Input: part model. Units: mm. Frame: model coordinates. Round coordinates to 2 decimals unless told otherwise and drop trailing zeros. Loops run counter-clockwise (first coordinate to the right, second up) from the corner with the lowest first, then second, coordinate; pieces in that order, holes last. Notation, with made-up numbers: M 58,-6 L 65,-6 A32 cw 65,27 Z; hole C 66,20 d7. An arc over 180 degrees is marked long. Use one line per item in the form item = value. Start each with the question number.
Q1. Mould query, pull axis X, two halves, no side actions, for faces 1 (the flat face through (61, 31, 27)), 2 (the cylindrical face through (66.96, 32.88, 31.93)), 3 (the flat face through (61, 31, 37)). Classes: pulls with the +X half, pulls with the -X half, needs draft (parallel to the pull), parting line crosses it, or undercut.
Q2. Ray query, line 1 along Z through (x, y) = (57.5, 33.25); line 2 along Y through (x, z) = (59.25, 34.25); line 3 along X through (y, z) = (30.25, 30). Return the intervals inside material, ascending.
Q3. Section query A-A, the plane y = 31. Output: boundary loops of the cut face in (x, z).
Q4. Section query B-B, the plane x = 61. Output: boundary loops of the cut face in (y, z).
Q5. Section query D-D, the plane y = 35.75. Output: boundary loops of the cut face in (x, z), and give its area (3 significant figures).
Q6. Section query C-C, the plane z = 35.5. Output: boundary loops of the cut face in (x, y).
Q7. First-contact query: P1, Ø2, axis at x = 65, z = 34, coming from the +Y side. Flat tip, straight axial feed; report the tip coordinate or a pass-through.
```python
from build123d import *

# Parameters (mm, degrees)
CYLINDER005_R         = 6.25
CYLINDER005_DEPTH     = 10
TORUS_R               = 0.25
TORUS_ANGLE           = 290
TORUS_PLACEMENT_ANGLE = 125


with BuildPart() as power_butt:
    # Cylinder005 → Cylinder005 (new body)
    with BuildSketch(Plane(origin=(61, 31, 27), x_dir=(1, 0, 0), z_dir=(0, 0, 1))):
        Circle(CYLINDER005_R)
    extrude(amount=CYLINDER005_DEPTH)


with BuildPart() as power_button:
    # Torus → Torus (revolve)
    with BuildSketch(Plane.XZ):
        with Locations((3, 0)):
            Circle(TORUS_R)
    revolve(axis=Axis((0, 0, 0), (0, 0, 1)), revolution_arc=TORUS_ANGLE)


with BuildPart() as power_button_1:
    # Torus placement: moved
    add(power_button.part.moved(Location((61, 31, 37))).rotate(Axis((61, 31, 37), (0, 0, 1)), TORUS_PLACEMENT_ANGLE))

    # Fusion006: union power_butt
    add(power_butt.part)


solid = power_button_1.part
```
Results found:
q1.face_1 = needs draft
q1.face_2 = parting line crosses it
q1.face_3 = undercut
q2.line_1 = 27 to 37
q2.line_2 = 25 to 37
q2.line_3 = 54.8 to 67.2
q3.outline = M 54.75,27 L 67.25,27 L 67.25,37 L 64.25,37 A0.25 ccw 63.75,37 L 58.25,37 A0.25 ccw 57.75,37 L 54.75,37 Z
q4.outline = M 24.75,27 L 37.25,27 L 37.25,37 L 28.25,37 A0.25 ccw 27.75,37 L 24.75,37 Z
q5.outline = M 56.94,27 L 65.06,27 L 65.06,37 L 56.94,37 Z
q5.area = 81.2 mm²
q6.outline = C 61,31 d12.5
q7.P1 = 36.48
